Study the drawing (mm; zero at the part's minimum x, y, z) and answer. A direction names the side the tool comes from. Give positions to 0.01 mm unless a question says otherwise; leave off trailing zeros. Write each loop counter-clockwise with the first axis right and the second up, starting at its lowest first coordinate (ties: lowest second). Pieces come first, ordered by that corner, then holes. Notation, with made-up numbers: (22, -21.5) -> (54, -21.5) arc R26 cw to (54, 9.5) -> close; hole circle Ø5 at (81, -39.75). An arc over 180 degrees is marked (long way). Put each result on its own line as item: value. Start each with the question number.
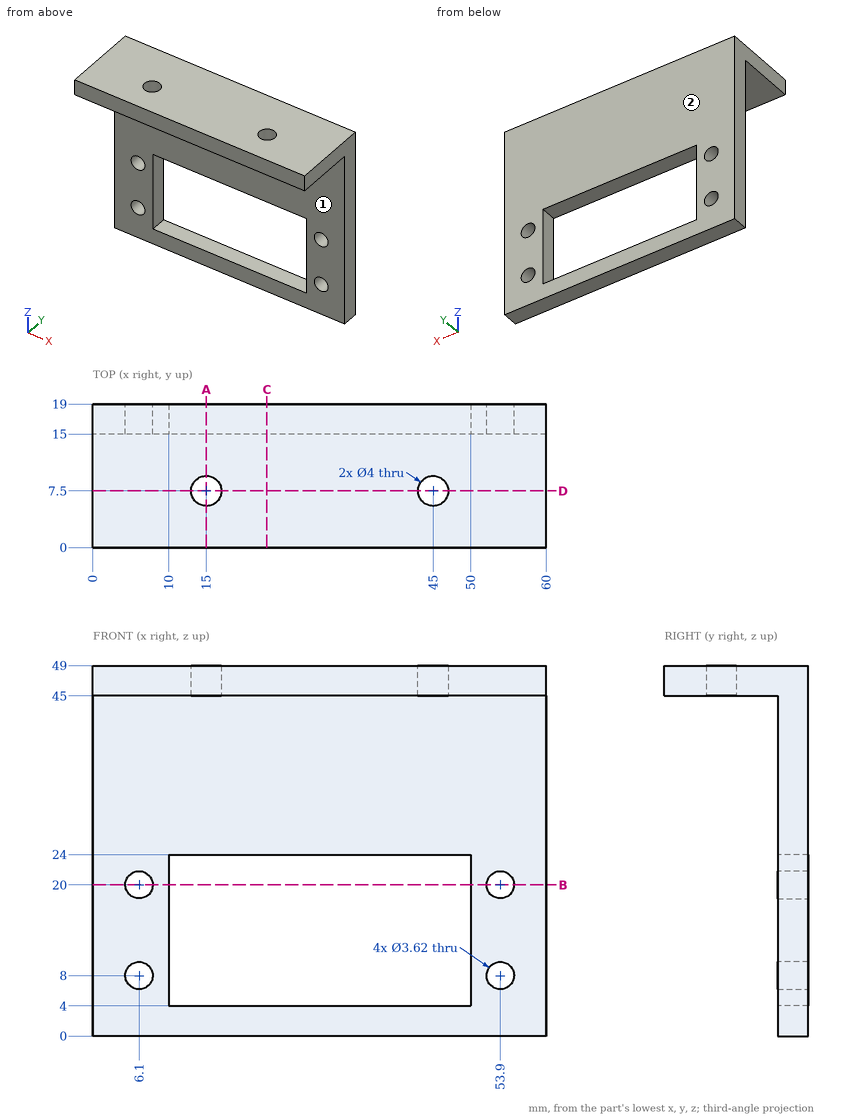
1) A cutting plane is placed at B-B on z = 20. Give the vertices of the cut face in (x, y), and give its area (3 significant figures).
2) A cutting plane is placed at C-C on x = 23. Give the vertices of the cut face in (y, z).
3) A cutting plane is placed at A-A on x = 15. Give the vertices of the cut face in (y, z), and give its area (3 significant figures).
4) Straight lines are drawn through the part: line 1 (X direction, y = 17.05, z = 20); line 2 (Z direction, x = 41, y = 16.5); line 3 (Y direction, x = 34, z = 35). For each, find the intervals that lie inside material, in ascending order. Write a range as [from, to].
5) A cutting plane is placed at D-D on y = 7.5. Give the vertices of the cut face in (x, z).
6) Each of these flat-tipped pins is pushed along its axis until it touches: pin 1 Ø6 at (x, z) = (53.9, 20) entering from +Y; pin 2 Ø12 at (x, z) = (28, 34) entering from -Y; pin 3 Ø8 at (x, y) = (18.5, 8) entering from -Z. Where does it stop, or does it pass through?
7) For the marked faces 1 and 2, determine the directions among +Z, -Z, +X, -X, +Y, -Y from which every point of the face is accessible in a straight line to the end or side of a thin tool.
Results found:
1. outline: (0, 15) -> (4.29, 15) -> (4.29, 19) -> (0, 19) -> close; (7.91, 15) -> (10, 15) -> (10, 19) -> (7.91, 19) -> close; (50, 15) -> (52.09, 15) -> (52.09, 19) -> (50, 19) -> close; (55.71, 15) -> (60, 15) -> (60, 19) -> (55.71, 19) -> close
1. area: 51.0 mm²
2. outline: (0, 45) -> (15, 45) -> (15, 24) -> (19, 24) -> (19, 49) -> (0, 49) -> close; (15, 0) -> (19, 0) -> (19, 4) -> (15, 4) -> close
3. outline: (0, 45) -> (5.5, 45) -> (5.5, 49) -> (0, 49) -> close; (9.5, 45) -> (15, 45) -> (15, 24) -> (19, 24) -> (19, 49) -> (9.5, 49) -> close; (15, 0) -> (19, 0) -> (19, 4) -> (15, 4) -> close
3. area: 160 mm²
4. line 1: x = [0, 4.29], [7.91, 10], [50, 52.09], [55.71, 60]
4. line 2: z = [0, 4], [24, 49]
4. line 3: y = [15, 19]
5. outline: (0, 45) -> (13, 45) -> (13, 49) -> (0, 49) -> close; (17, 45) -> (43, 45) -> (43, 49) -> (17, 49) -> close; (47, 45) -> (60, 45) -> (60, 49) -> (47, 49) -> close
6. pin 1: stops at y = 19
6. pin 2: stops at y = 15
6. pin 3: stops at z = 45
7. face 1: -Z, +X, -X, -Y
7. face 2: +Z, -Z, +X, -X, +Y
